The drawing under review shows one solid part. Ordinate dimensions are in mm from its lowest x, y, z. A direction names the side the tool comes from. Round coordinates to 2 decimals unless told otherwise and drop trailing zeros. Write each loop counter-clockwise with the first axis right and the second up, starting at its lowest first coordinate (ties: lowest second). Pieces come first, ordered by that corner, then holes. Notation, with made-up numbers: (52.5, 41) -> (60.5, 41) arc R22 ccw to (60.5, 50) -> close; hole circle Ø7 at (45.25, 2). An arc over 180 degrees is marked (long way). Write item = value, one per line. Start each with the question number.
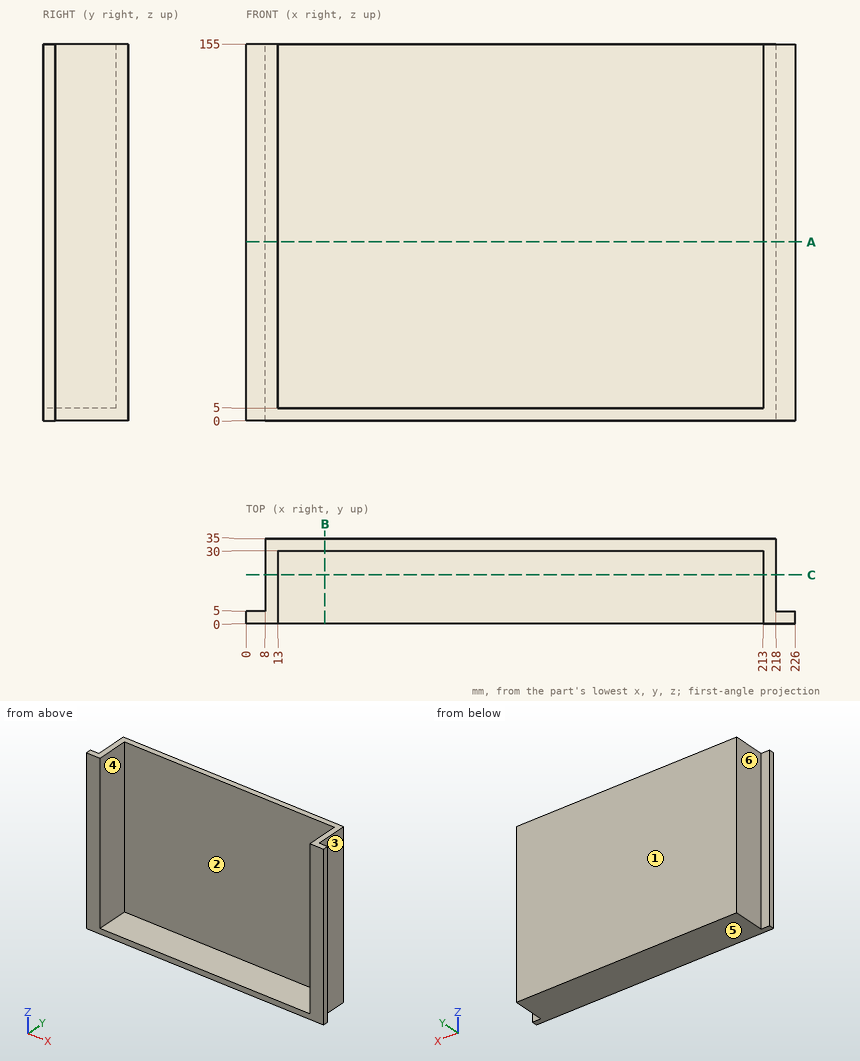
1. Consider section C-C, the plane y = 20. Give the boundary of the cut face in (x, z).
2. Draft analysis for pull direction X (two halves, no side actions). For the marked faces 4, 5 and 6, state which applies: +X half, -X half, draft (parallel to the pull), parting line (faces both ways), or undercut.
3. Clearance check with flat-ended pins moving along their axes: pin 1 Ø8 at (y, z) = (25, 51.5) entering from -X; pin 2 Ø1.5 at (y, z) = (25, 32.5) entering from +X; pin 3 Ø2.5 at (x, z) = (2, 101.5) entering from +Y. State where each tip first meets the part, or that it passes through.
4. Consider section B-B, the plane x = 32.5. Give the boundary of the cut face in (y, z).
5. Machinability: for the marked faces 1, 2 and 3, which of the approach directions +Z, -Z, +X, -X, +Y, -Y give a long, thin tool a straight path to every point of the face, cutting with its end or side? Answer none if there is none.
6. Consider section A-A, the plane z = 73.5. Give the boundary of the cut face in (x, y), then the cut area to 3 significant figures.
7. Wall thickness on L1, parallel to X at y = 12.5, z = 124; L2, parallel to X at y = 1.5, z = 21.5; L3, parallel to Y at x = 104, z = 79: over which ranges is each line inside the solid? List them lowest first. Write a range as from..to.
Outcome:
q1.outline = (8, 0) -> (218, 0) -> (218, 155) -> (213, 155) -> (213, 5) -> (13, 5) -> (13, 155) -> (8, 155) -> close
q2.face_4 = undercut
q2.face_5 = draft
q2.face_6 = -X half
q3.pin_1 = 8
q3.pin_2 = 218
q3.pin_3 = 5
q4.outline = (0, 0) -> (35, 0) -> (35, 155) -> (30, 155) -> (30, 5) -> (0, 5) -> close
q5.face_1 = +Z, -Z, +X, -X, +Y
q5.face_2 = +Z, -Y
q5.face_3 = +Z, -Z, +X, +Y
q6.outline = (0, 0) -> (13, 0) -> (13, 30) -> (213, 30) -> (213, 0) -> (226, 0) -> (226, 5) -> (218, 5) -> (218, 35) -> (8, 35) -> (8, 5) -> (0, 5) -> close
q6.area = 1,430 mm2
q7.L1 = 8..13, 213..218
q7.L2 = 0..13, 213..226
q7.L3 = 30..35
